Here's how the part is built. I have some questions about the finished solid (model axes, mm). Coordinates: 2 decimals unless noted, no trailing zeros. Loops run counter-clockwise (first coordinate to the right, second up) from the corner with the lowest first, then second, coordinate; pieces in that order, holes last. Notation, with made-up numbers: M 60,-6 L 96,-6 A33 ccw 96,23 Z; hole C 49.25,-12.75 d7. An arc over 180 degrees is marked long. Use CSV: the item, a comma, the result in double quotes. Start each with the question number.
Q1. If we section it at B-B (y = 1.5): State how many separate pieces and enclosed holes the cut face has, and give its area (3 significant figures).
Q2. Please list where these lines run through material, in increasing order: probe 1 along X at (y, z) = (1, 0); probe 2 along X at (y, z) = (2.5, 130); probe 3 along Z at (x, y) = (194, -0.25). Write a range as [from, to].
Q3. If we section it at A-A (z = 122): Please give me the cut outline in (x, y), and give its area (3 significant figures).
Q4. For pin 1 Ø2.5 at (x, z) = (-194, -125) entering from +Y, with a flat end and sliding along its axis, tell me the tip position at first contact or that it passes through.
from build123d import *

# Parameters (mm, degrees)
SKETCH1_W             = 420
SKETCH1_H             = 300
BOSS_EXTRUDE1_DEPTH   = 4
CHAMFER1_SIZE         = 3
M8_TAPPED_HOLE1_D     = 6.8
M8_TAPPED_HOLE1_DEPTH = 19.75
M8_TAPPED_HOLE1_TIP   = 2.042926105
M5_TAPPED_HOLE1_D     = 4.2
M5_TAPPED_HOLE1_DEPTH = 12.4
M5_TAPPED_HOLE1_TIP   = 1.2618073
SKETCH6_W             = 139.582677991
SKETCH6_H             = 303.771276781
CUT_EXTRUDE1_DEPTH    = 10


with BuildPart() as part:
    # Sketch1 → Boss-Extrude1 (new, symmetric)
    with BuildSketch(Plane(origin=(0, 0, 0), x_dir=(1, 0, 0), z_dir=(0, 1, 0))):
        Rectangle(SKETCH1_W, SKETCH1_H)
    extrude(amount=BOSS_EXTRUDE1_DEPTH, both=True)

    # Chamfer1
    chamfer1_edges = [part.edges().sort_by_distance(p)[0] for p in [
        (210, 0, 150),
        (-210, 0, 150),
        (-210, 0, -150),
        (210, 0, -150),
    ]]
    chamfer(chamfer1_edges, length=CHAMFER1_SIZE)

    # M8 Tapped Hole1
    with Locations(Plane(origin=(-190, 4, -80), x_dir=(0, 0, 1), z_dir=(0, 1, 0))):
        with Locations((0, 0), (0, 206), (80, 206), (80, 0), (48, 246), (48, 376), (3, 376), (3, 246)):
            Hole(M8_TAPPED_HOLE1_D / 2, depth=M8_TAPPED_HOLE1_DEPTH)
            with Locations((0, 0, -(M8_TAPPED_HOLE1_DEPTH + M8_TAPPED_HOLE1_TIP / 2))):  # 118° drill point
                Cone(0, M8_TAPPED_HOLE1_D / 2, M8_TAPPED_HOLE1_TIP, mode=Mode.SUBTRACT)

    # M5 Tapped Hole1
    with Locations(Plane(origin=(0, 4, 0), x_dir=(-1, 0, 0), z_dir=(0, 1, 0))):
        with Locations((175, 130), (-175, 130), (-175, -130), (175, -130), (194, -125), (194, 55), (-194, 55), (-194, -125), (174.5, 66), (174.5, 36), (-0.5, 36), (-0.5, 66)):
            Hole(M5_TAPPED_HOLE1_D / 2, depth=M5_TAPPED_HOLE1_DEPTH)
            with Locations((0, 0, -(M5_TAPPED_HOLE1_DEPTH + M5_TAPPED_HOLE1_TIP / 2))):  # 118° drill point
                Cone(0, M5_TAPPED_HOLE1_D / 2, M5_TAPPED_HOLE1_TIP, mode=Mode.SUBTRACT)

    # Sketch6 → Cut-Extrude1 (cut)
    with BuildSketch(Plane(origin=(0, 4, 0), x_dir=(1, 0, 0), z_dir=(0, 1, 0))):
        with Locations((-90.81821677, -11.184509455)):
            Rectangle(SKETCH6_W, SKETCH6_H)
    extrude(amount=-CUT_EXTRUDE1_DEPTH, mode=Mode.SUBTRACT)


solid = part.part
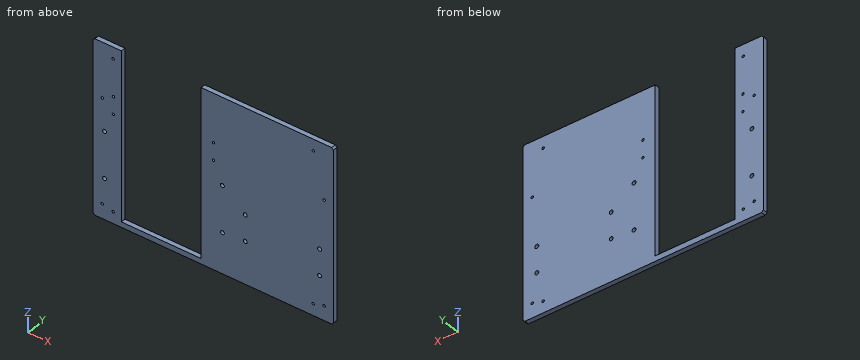
Results below:
1,separate pieces,"1"
1,enclosed holes,"20"
1,area,"84,900 mm^2"
2,probe 1,"[-210, -193.4], [-186.6, -160.61], [-21.03, 12.6], [19.4, 210]"
2,probe 2,"[-210, -177.1], [-172.9, -160.61], [-21.03, 172.9], [177.1, 210]"
2,probe 3,"[-150, -127.1], [-122.9, 52.9], [57.1, 150]"
3,outline,"M -210,-4 L -160.61,-4 L -160.61,4 L -210,4 Z; M -21.03,-4 L 210,-4 L 210,4 L -21.03,4 Z"
3,area,"2,240 mm^2"
4,pin 1,"through"
